from build123d import *

# Parameters (mm, degrees)
SKETCH_1_W                = 270
SKETCH_1_H                = 40
EXTRUDE_1_DEPTH           = 15
HOLE_WIZARD_1_D           = 13.5
HOLE_WIZARD_1_CBORE_D     = 20
HOLE_WIZARD_1_CBORE_DEPTH = 12.2
CUT_EXTRUDE_1_DEPTH       = 138.295302177
HOLE_WIZARD_M8_1_D        = 6.8
HOLE_WIZARD_1_2_D         = 8


with BuildPart() as part:
    # 草图1 → 凸台-拉伸1 (new body)
    with BuildSketch(Plane.XY):
        Rectangle(SKETCH_1_W, SKETCH_1_H)
    extrude(amount=EXTRUDE_1_DEPTH)

    # Hole Wizard 1 (through all)
    with Locations(Plane(origin=(0, 0, 0), x_dir=(-1, 0, 0), z_dir=(0, 0, -1))):
        with Locations((-82, 0), (82, 0)):
            CounterBoreHole(HOLE_WIZARD_1_D / 2, HOLE_WIZARD_1_CBORE_D / 2, HOLE_WIZARD_1_CBORE_DEPTH)

    # 草图4 → 切除-拉伸1 (cut, through all)
    with BuildSketch(Plane.XY.offset(15)):
        with BuildLine():
            ThreePointArc((114.867278915, -12.073037507), (115.5, 0), (114.867278915, 12.073037507))
            ThreePointArc((114.867278915, 12.073037507), (118.872249359, 17.018764121), (123.817975973, 13.013793677))
            ThreePointArc((123.817975973, 13.013793677), (124.5, 0), (123.817975973, -13.013793677))
            ThreePointArc((123.817975973, -13.013793677), (118.872249359, -17.018764121), (114.867278915, -12.073037507))
        make_face()
        with BuildLine():
            ThreePointArc((-114.867278915, -12.073037507), (-118.872249359, -17.018764121), (-123.817975973, -13.013793677))
            ThreePointArc((-123.817975973, -13.013793677), (-124.5, 0), (-123.817975973, 13.013793677))
            ThreePointArc((-123.817975973, 13.013793677), (-118.872249359, 17.018764121), (-114.867278915, 12.073037507))
            ThreePointArc((-114.867278915, 12.073037507), (-115.5, 0), (-114.867278915, -12.073037507))
        make_face()
    extrude(amount=-CUT_EXTRUDE_1_DEPTH, mode=Mode.SUBTRACT)

    # M8 螺纹孔1 (through all)
    with Locations(Plane.XY.offset(15)):
        with Locations((-37, 0), (37, 0)):
            Hole(HOLE_WIZARD_M8_1_D / 2)

    # Hole Wizard 1 2 (through all)
    with Locations(Plane(origin=(0, 0, 0), x_dir=(-1, 0, 0), z_dir=(0, 0, -1))):
        with Locations((0, 0)):
            Hole(HOLE_WIZARD_1_2_D / 2)


solid = part.part
Verification items for the finished model (mm, model axes). A direction names the side the tool comes from. Coordinates: 2 decimals unless noted, no trailing zeros. Order: outer loops, then holes, each group sorted by start corner. A loop starts at its lowest first (then second) coordinate and runs counter-clockwise, first axis right, second up.
1. Set-up check for faces 1 (the face through (92, 0, 6)), 2 (the face through (-2, -4, 0)), 3 (the face through (-118.971, 17.028, 7.605)): record each of +Z, -Z, +X, -X, +Y, -Y from which the full face is reachable in a straight line by a thin tool's end or side.
Results found:
face 1: -Z
face 2: -Z, +X, -X, +Y, -Y
face 3: +Z, -Z
2. Sectioned sample at B-B, the plane z = 6.25. Record the cut outline in (x, y).
Results found:
outline: (-135, -20) - (135, -20) - (135, 20) - (-135, 20) - close; hole (-123.82, -13.01) arc R4.5 ccw to (-114.87, -12.07) arc R115.5 cw to (-114.87, 12.07) arc R4.5 ccw to (-123.82, 13.01) arc R124.5 ccw to start; hole circle Ø20 at (-82, 0); hole circle Ø6.8 at (-37, 0); hole circle Ø8 at (0, 0); hole circle Ø6.8 at (37, 0); hole circle Ø20 at (82, 0); hole (114.87, -12.07) arc R4.5 ccw to (123.82, -13.01) arc R124.5 ccw to (123.82, 13.01) arc R4.5 ccw to (114.87, 12.07) arc R115.5 cw to start
3. Sectioned sample at D-D, the plane x = -82. Record the cut outline in (y, z).
Results found:
outline: (-20, 0) - (-10, 0) - (-10, 12.2) - (-6.75, 12.2) - (-6.75, 15) - (-20, 15) - close; (6.75, 12.2) - (10, 12.2) - (10, 0) - (20, 0) - (20, 15) - (6.75, 15) - close
4. Sectioned sample at A-A, the plane x = -37. Record the cut outline in (y, z).
Results found:
outline: (-20, 0) - (-3.4, 0) - (-3.4, 15) - (-20, 15) - close; (3.4, 0) - (20, 0) - (20, 15) - (3.4, 15) - close
5. Go/stop test with flat-tipped pins: pin 1 Ø6 at (x, y) = (-37, 0) entering from +Z; pin 2 Ø18 at (x, y) = (-82, 0) entering from -Z. Record where each tip stops, or that it passes through.
Results found:
pin 1: passes through
pin 2: stops at z = 12.2
6. Scan lines: line 1 (Y direction, x = -119.5, z = 4.5); line 2 (X direction, y = 9, z = 5.5); line 3 (Y direction, x = 82, z = 13.55). Record each from-to range of solid material in increasing order.
Results found:
line 1: y = -20 to -17.04, 17.04 to 20
line 2: x = -135 to -124.17, -115.15 to -86.36, -77.64 to 77.64, 86.36 to 115.15, 124.17 to 135
line 3: y = -20 to -6.75, 6.75 to 20
7. Sectioned sample at C-C, the plane y = 0. Give the number of separate pieces and of enclosed holes in the cut face, and give its area (3 significant figures).
Results found:
separate pieces: 8
enclosed holes: 0
area: 2,890 mm2
8. Release check for a two-part mould opening along Y. For faces 4 (the face through (118.971, -17.028, 7.605)), 5 (the face through (-135, 0, 7)), 6 (the face through (-2, -20, 7)) record: +Y half, -Y half, draft (parallel to the pull), parting line (faces both ways), or undercut.
Results found:
face 4: undercut
face 5: draft
face 6: -Y half
